The listing builds one solid part. Answer for the finished solid, in the listing's coordinates (mm). A direction names the side the tool comes from. Coordinates: 2 decimals unless noted, no trailing zeros. Loops run counter-clockwise (first coordinate to the right, second up) from the corner with the lowest first, then second, coordinate; pieces in that order, holes last. Notation, with made-up numbers: M 46.25,20.5 L 84.25,20.5 A8 ccw 84.25,29.5 Z; hole C 38,42 d8. An arc over 180 degrees is marked long. Answer as a JSON object with one key per item and string values. Group by question number.
1. A cutting plane is placed at A-A on x = -12.5. Give the vertices of the cut face in (y, z), and give its area (3 significant figures).
2. Given pin 1 (2 mm diameter, centred on y = -36.5, z = 28, fed in from +X); pin 2 (12.5 mm diameter, centred on x = -11, z = 26, fed in from +Y); pin 3 (7.5 mm diameter, centred on y = 11.5, z = 24, fed in from +X), each flat-ended and moving along its own axis, determine where each tip first touches the part or whether it passes through.
3. Determine the mould class of faces 1 (the face through (-1, 45.731, 6)), 2 (the face through (-64.27, -1, 6)), 3 (the face through (-1, 0, 12.7)) for opening direction X: released by +X, released by -X, zero draft, split by the parting line, or undercut.
4. A cutting plane is placed at C-C on y = -25. Give the vertices of the cut face in (x, z), and give its area (3 significant figures).
5. Straight lines are drawn through the part: L1, parallel to Z at x = -17.5, y = 26; L2, parallel to Z at x = -52, y = 7.5; L3, parallel to X at y = -20, z = 23.5. For each, find the intervals that lie inside material, in ascending order.
6. For faces 4 (the face through (38.706, 0, 26)), 5 (the face through (-1, -1, 0.508)), 6 (the face through (64.27, -1, 6)), determine the directions among +Z, -Z, +X, -X, +Y, -Y from which every point of the face is accessible in a straight line to the end or side of a thin tool.
7. A cutting plane is placed at B-B on z = 17. Give the vertices of the cut face in (x, y).
8. A cutting plane is placed at D-D on z = 35. Give the vertices of the cut face in (x, y), and give its area (3 significant figures).
from build123d import *

# Parameters (mm, degrees)
F0_W      = 128.5392045975
F0_H      = 91.4615094662
F1_DEPTH  = 12.7
F1_FACE_W = 128.5392045975
F1_FACE_H = 91.4615094662
F2_DEPTH  = 25.4
F2_TAPER  = 25
F3_W      = 128.0312045975
F3_H      = 90.9535094662
F4_DEPTH  = 0.508
F5_W      = 77.4115473032
F5_H      = 55.2224069834
F6_DEPTH  = 25.4
F7_R      = 2.4747052008
F8_DEPTH  = 45.573990792


with BuildPart() as f1:
    # F0 (on Top) → F1 (new body)
    with BuildSketch(Plane.XY):
        Rectangle(F0_W, F0_H)
    extrude(amount=F1_DEPTH)

    # F1_face (on face) → F2 (join)
    with BuildSketch(Plane.XY.offset(12.7)):
        Rectangle(F1_FACE_W, F1_FACE_H)
    extrude(amount=F2_DEPTH, taper=F2_TAPER)

    # F3 (on face) → F4 (cut)
    with BuildSketch(Plane(origin=(0, 0, 0), x_dir=(1, 0, 0), z_dir=(0, 0, -1))):
        Rectangle(F3_W, F3_H)
    extrude(amount=-F4_DEPTH, mode=Mode.SUBTRACT)

    # F5 (on face) → F6 (cut)
    with BuildSketch(Plane.XY.offset(38.1)):
        Rectangle(F5_W, F5_H)
    extrude(amount=-F6_DEPTH, mode=Mode.SUBTRACT)

    # F7 (on face) → F8 (cut)
    with BuildSketch(Plane.XY.offset(12.7)):
        with Locations((-34.4637036324, 23.5804095864)):
            Circle(F7_R)
    extrude(amount=-F8_DEPTH, mode=Mode.SUBTRACT)


solid = f1.part
From the geometry:
{
 "1": {"outline": "M -45.73,0 L -45.48,0 L -45.48,0.51 L 45.48,0.51 L 45.48,0 L 45.73,0 L 45.73,12.7 L 33.89,38.1 L 27.61,38.1 L 27.61,12.7 L -27.61,12.7 L -27.61,38.1 L -33.89,38.1 L -45.73,12.7 Z", "area": "1,730 mm²"},
 "2": {"pin 1": "stops at x = 57.6", "pin 2": "stops at y = 42.44", "pin 3": "stops at x = 60.75"},
 "3": {"face 1": "zero draft", "face 2": "released by -X", "face 3": "undercut"},
 "4": {"outline": "M -64.27,0 L -64.02,0 L -64.02,0.51 L 64.02,0.51 L 64.02,0 L 64.27,0 L 64.27,12.7 L 52.43,38.1 L 38.71,38.1 L 38.71,12.7 L -38.71,12.7 L -38.71,38.1 L -52.43,38.1 L -64.27,12.7 Z", "area": "2,570 mm²"},
 "5": {"L1": "z = 0.51 to 12.7", "L2": "z = 0.51 to 38.1", "L3": "x = -59.23 to -38.71, 38.71 to 59.23"},
 "6": {"face 4": "+Z", "face 5": "-Z", "face 6": "+Z, -Z, +X, +Y, -Y"},
 "7": {"outline": "M -62.26,-43.73 L 62.26,-43.73 L 62.26,43.73 L -62.26,43.73 Z; hole M -38.71,-27.61 L 38.71,-27.61 L 38.71,27.61 L -38.71,27.61 Z"},
 "8": {"outline": "M -53.87,-35.33 L 53.87,-35.33 L 53.87,35.33 L -53.87,35.33 Z; hole M -38.71,-27.61 L 38.71,-27.61 L 38.71,27.61 L -38.71,27.61 Z", "area": "3,340 mm²"}
}
